```python
from build123d import *

# Parameters (mm, degrees)
SKETCH_1_W          = 170
SKETCH_1_H          = 60
EXTRUDE_1_DEPTH     = 5
SKETCH_2_W          = 150
SKETCH_2_H          = 40
CUT_EXTRUDE_1_DEPTH = 5
SKETCH_3_W          = 8
SKETCH_3_H          = 40
EXTRUDE_2_DEPTH     = 5
FILLET_1_R          = 3
FILLET_2_R          = 2
SKETCH_4_R          = 1.525
CUT_EXTRUDE_2_DEPTH = 5


with BuildPart() as part:
    # 草图1 → 凸台-拉伸1 (new body)
    with BuildSketch(Plane.XY):
        Rectangle(SKETCH_1_W, SKETCH_1_H)
    extrude(amount=EXTRUDE_1_DEPTH)

    # 草图2 → 切除-拉伸1 (cut)
    with BuildSketch(Plane.XY.offset(5)):
        Rectangle(SKETCH_2_W, SKETCH_2_H)
    extrude(amount=-CUT_EXTRUDE_1_DEPTH, mode=Mode.SUBTRACT)

    # 草图3 → 凸台-拉伸2 (add)
    with BuildSketch(Plane.XY.offset(5)):
        Rectangle(SKETCH_3_W, SKETCH_3_H)
    extrude(amount=-EXTRUDE_2_DEPTH)

    # 圆角1
    fillet_1_edges = [part.edges().sort_by_distance(p)[0] for p in [
        (85, -30, 2.5),
        (-85, -30, 2.5),
        (-85, 30, 2.5),
        (85, 30, 2.5),
    ]]
    fillet(fillet_1_edges, radius=FILLET_1_R)

    # 圆角2
    fillet_2_edges = [part.edges().sort_by_distance(p)[0] for p in [
        (75, 20, 2.5),
        (75, -20, 2.5),
        (-75, -20, 2.5),
        (-75, 20, 2.5),
        (-4, 20, 2.5),
        (-4, -20, 2.5),
        (4, -20, 2.5),
        (4, 20, 2.5),
    ]]
    fillet(fillet_2_edges, radius=FILLET_2_R)

    # 草图4 → 切除-拉伸2 (cut)
    with BuildSketch(Plane(origin=(0, 0, 0), x_dir=(-1, 0, 0), z_dir=(0, 0, -1))):
        with Locations((80, 20)):
            Circle(SKETCH_4_R)
        with Locations((80, 0)):
            Circle(SKETCH_4_R)
        with Locations((0, -20)):
            Circle(SKETCH_4_R)
        with Locations((0, 20)):
            Circle(SKETCH_4_R)
        with Locations((-80, 20)):
            Circle(SKETCH_4_R)
        with Locations((-80, 0)):
            Circle(SKETCH_4_R)
        with Locations((-80, -20)):
            Circle(SKETCH_4_R)
        Circle(SKETCH_4_R)
        with Locations((80, -20)):
            Circle(SKETCH_4_R)
    extrude(amount=-CUT_EXTRUDE_2_DEPTH, mode=Mode.SUBTRACT)


solid = part.part
```
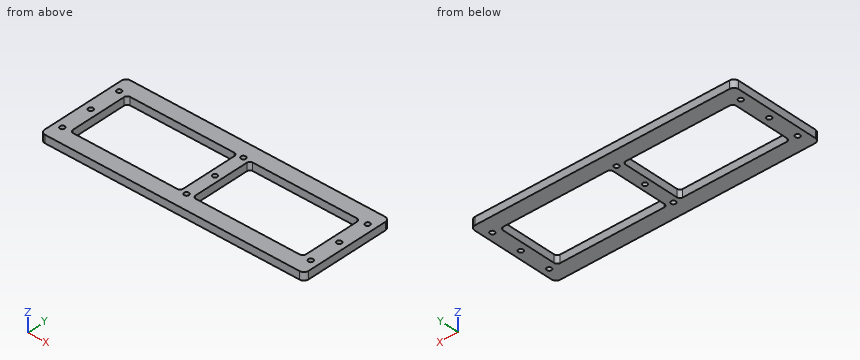
Work out the finished part from the listing and answer in its coordinate system (mm). Round coordinates to 2 decimals unless told otherwise and drop trailing zeros. Write each loop counter-clockwise with the first axis right and the second up, starting at its lowest first coordinate (ties: lowest second). Pieces come first, ordered by that corner, then holes. Notation, with made-up numbers: (59.5, 1) -> (100.5, 1) arc R14 cw to (100.5, 22) -> close; hole circle Ø3 at (32, 49.5). An arc over 180 degrees is marked (long way). Write each question's results on one line, items separated by ' | '.
1) The part is cut by section C-C (y = 12.5). Write down the section's boundary in (x, z).
Findings:
outline: (-85, 0) -> (-75, 0) -> (-75, 5) -> (-85, 5) -> close; (-4, 0) -> (4, 0) -> (4, 5) -> (-4, 5) -> close; (75, 0) -> (85, 0) -> (85, 5) -> (75, 5) -> close
2) The part is cut by section B-B (z = 0.75). State how many separate pieces and enclosed holes the cut face has, and give its area (3 significant figures).
Findings:
separate pieces: 1 | enclosed holes: 11 | area: 4,450 mm²
3) The part is cut by section A-A (x = 68). Write down the section's boundary in (y, z), and give its area (3 significant figures).
Findings:
outline: (-30, 0) -> (-20, 0) -> (-20, 5) -> (-30, 5) -> close; (20, 0) -> (30, 0) -> (30, 5) -> (20, 5) -> close | area: 100 mm²
4) Consider line 1 along Y through (x, z) = (-80, 1.05) (3 decimals); line 2 along X through (y, z) = (-6, 4.05); line 3 along Y through (x, z) = (-69.5, 3.4). Determine where each line is inside the solid, lowest interval first. Write a range as [from, to].
Findings:
line 1: y = [-30, -21.525], [-18.475, -1.525], [1.525, 18.475], [21.525, 30] | line 2: x = [-85, -75], [-4, 4], [75, 85] | line 3: y = [-30, -20], [20, 30]
